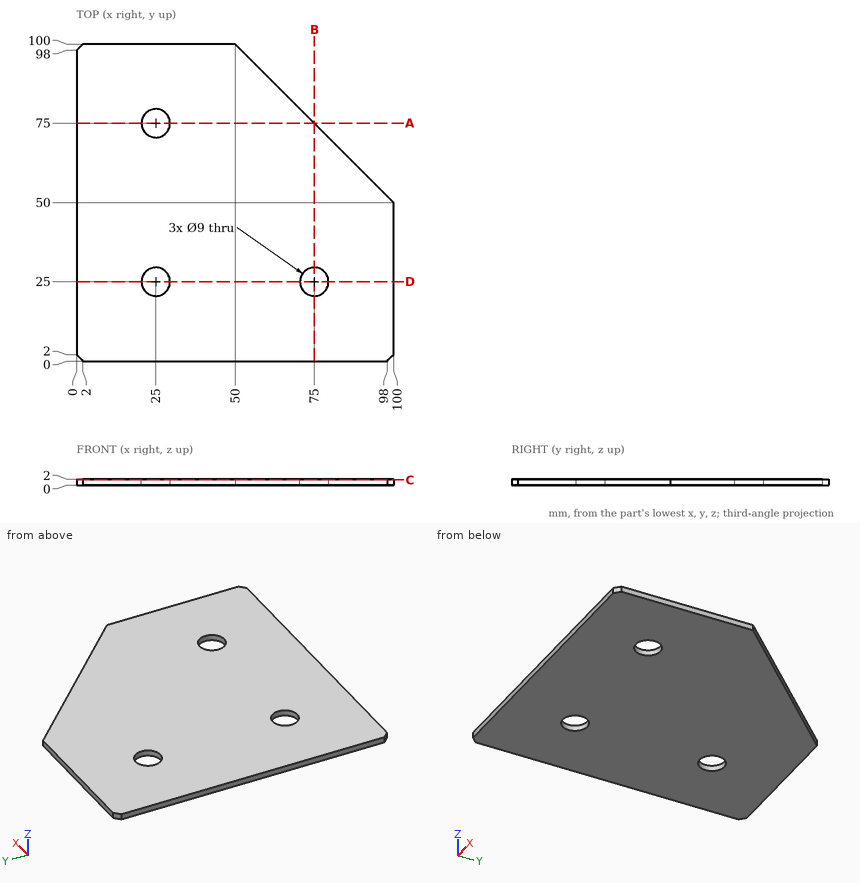
Verification items for this drawing (mm, ordinates from the low corner). Coordinates: 2 decimals unless noted, no trailing zeros. Write each loop counter-clockwise with the first axis right and the second up, starting at its lowest first coordinate (ties: lowest second). Pieces come first, ordered by that corner, then holes. Notation, with made-up numbers: (7, -25.75) -> (37, -25.75) arc R11 cw to (37, -14.75) -> close; hole circle Ø4 at (50.5, 26). An arc over 180 degrees is marked (long way). One line per item, written item: value. Start each with the question number.
Q1. Go/stop test with a flat-tipped pin: P1, Ø7, axis at x = 25, y = 75, coming from the +Z side. Record where the tip stops, or that it passes through.
Q2. Cross-section at A-A on y = 75. Enter the section's corners in (x, z).
Q3. Cross-section at C-C on z = 1.7. Enter the section's corners in (x, y).
Q4. Cross-section at D-D on y = 25. Enter the section's corners in (x, z).
Q5. Thickness scan on L1, parallel to Y at x = 25.5, z = 0.4; L2, parallel to X at y = 25, z = 1.4; L3, parallel to X at y = 29, z = 0.2. Record the ranges inside material, lowest first. Write a range as from..to.
Checked values:
1. P1: passes through
2. outline: (0, 0) -> (20.5, 0) -> (20.5, 2) -> (0, 2) -> close; (29.5, 0) -> (75, 0) -> (75, 2) -> (29.5, 2) -> close
3. outline: (0, 2) -> (2, 0) -> (98, 0) -> (100, 2) -> (100, 50) -> (50, 100) -> (2, 100) -> (0, 98) -> close; hole circle Ø9 at (25, 25); hole circle Ø9 at (25, 75); hole circle Ø9 at (75, 25)
4. outline: (0, 0) -> (20.5, 0) -> (20.5, 2) -> (0, 2) -> close; (29.5, 0) -> (70.5, 0) -> (70.5, 2) -> (29.5, 2) -> close; (79.5, 0) -> (100, 0) -> (100, 2) -> (79.5, 2) -> close
5. L1: y = 0..20.53, 29.47..70.53, 79.47..100
5. L2: x = 0..20.5, 29.5..70.5, 79.5..100
5. L3: x = 0..22.94, 27.06..72.94, 77.06..100
